Input: part model. Units: mm. Frame: model coordinates. A direction names the side the tool comes from. Give positions to 0.01 mm unless a question says otherwise; leave off trailing zeros. Write each loop counter-clockwise with the first axis right and the second up, starting at its lowest first coordinate (ties: lowest second). Pieces come first, ordered by that corner, then holes.
```python
from build123d import *

# Parameters (mm, degrees)
EXTRUDE_2_DEPTH     = 8
SKETCH_4_R          = 3.5
SKETCH_4_R_2        = 8.462893534
CUT_EXTRUDE_1_DEPTH = 126.60827275


with BuildPart() as part:
    # 草图1 → 凸台-拉伸2 (new body)
    with BuildSketch(Plane.XY):
        with BuildLine():
            ThreePointArc((-44.271832455, 12.900159535), (-42.760990151, 12.93891125), (-41.460762065, 13.709335217))
            ThreePointArc((-41.460762065, 13.709335217), (-27.63735599, 19.468755163), (-13.813949915, 13.709335217))
            ThreePointArc((-13.813949915, 13.709335217), (-12.513721829, 12.93891125), (-11.002879525, 12.900159535))
            Line((-11.002879525, 12.900159535), (59.529347881, 29.339622898))
            ThreePointArc((59.529347881, 29.339622898), (61.75543851, 28.989437599), (63.109724345, 27.188321525))
            Line((63.109724345, 27.188321525), (66.427142402, 14.703033787))
            ThreePointArc((66.427142402, 14.703033787), (65.985368626, 12.212155416), (63.796050229, 10.944668104))
            Line((63.796050229, 10.944668104), (-5.503908774, 4.721894109))
            ThreePointArc((-5.503908774, 4.721894109), (-7.526265644, 3.671148438), (-8.226657796, 1.502405805))
            ThreePointArc((-8.226657796, 1.502405805), (-8.168778443, 0.083161809), (-8.214531044, -1.33652486))
            ThreePointArc((-8.214531044, -1.33652486), (-7.503974356, -3.489473399), (-5.489913373, -4.530452062))
            Line((-5.489913373, -4.530452062), (63.846058336, -10.75645981))
            ThreePointArc((63.846058336, -10.75645981), (66.035376732, -12.023947122), (66.477150508, -14.514825493))
            Line((66.477150508, -14.514825493), (63.142843844, -27.063674443))
            ThreePointArc((63.142843844, -27.063674443), (61.732433193, -28.897690671), (59.436427456, -29.182701869))
            Line((59.436427456, -29.182701869), (-8.561409136, -10.190770239))
            ThreePointArc((-8.561409136, -10.190770239), (-10.364737659, -10.250456004), (-11.807672821, -11.33373541))
            ThreePointArc((-11.807672821, -11.33373541), (-27.63735599, -19.468755163), (-43.467039159, -11.33373541))
            ThreePointArc((-43.467039159, -11.33373541), (-44.909974321, -10.250456004), (-46.713302844, -10.190770239))
            Line((-46.713302844, -10.190770239), (-114.711139436, -29.182701869))
            ThreePointArc((-114.711139436, -29.182701869), (-117.007145173, -28.897690671), (-118.417555824, -27.063674443))
            Line((-118.417555824, -27.063674443), (-121.751862488, -14.514825493))
            ThreePointArc((-121.751862488, -14.514825493), (-121.310088712, -12.023947122), (-119.120770315, -10.75645981))
            Line((-119.120770315, -10.75645981), (-49.784798606, -4.530452062))
            ThreePointArc((-49.784798606, -4.530452062), (-47.770737623, -3.489473399), (-47.060180936, -1.33652486))
            ThreePointArc((-47.060180936, -1.33652486), (-47.105933537, 0.083161809), (-47.048054184, 1.502405805))
            ThreePointArc((-47.048054184, 1.502405805), (-47.748446336, 3.671148438), (-49.770803206, 4.721894109))
            Line((-49.770803206, 4.721894109), (-119.070762209, 10.944668104))
            ThreePointArc((-119.070762209, 10.944668104), (-121.260080606, 12.212155416), (-121.701854382, 14.703033787))
            Line((-121.701854382, 14.703033787), (-118.384436325, 27.188321525))
            ThreePointArc((-118.384436325, 27.188321525), (-117.03015049, 28.989437599), (-114.804059861, 29.339622898))
            Line((-114.804059861, 29.339622898), (-44.271832455, 12.900159535))
        make_face()
    extrude(amount=EXTRUDE_2_DEPTH)

    # 草图4 → 切除-拉伸1 (cut, through all)
    with BuildSketch(Plane.XY.offset(8)):
        with Locations((-115.63735599, -20)):
            Circle(SKETCH_4_R)
        with Locations((-115.63735599, 20)):
            Circle(SKETCH_4_R)
        with Locations((60.36264401, -20)):
            Circle(SKETCH_4_R)
        with Locations((60.36264401, 20)):
            Circle(SKETCH_4_R)
        with Locations((-27.63735599, 0)):
            Circle(SKETCH_4_R_2)
        with BuildLine():
            ThreePointArc((-37.984908909, -8.703484854), (-35.348611937, -6.039852319), (-38.012244471, -3.403555348))
            ThreePointArc((-38.012244471, -3.403555348), (-40.648541443, -6.067187882), (-37.984908909, -8.703484854))
        make_face()
        with BuildLine():
            ThreePointArc((-25.273693465, -13.312986121), (-26.26231842, -9.698069705), (-29.877234836, -10.68669466))
            ThreePointArc((-29.877234836, -10.68669466), (-28.888609881, -14.301611076), (-25.273693465, -13.312986121))
        make_face()
        with BuildLine():
            ThreePointArc((-19.502346355, -7.283139312), (-15.877424428, -8.234423195), (-14.926140546, -4.609501268))
            ThreePointArc((-14.926140546, -4.609501268), (-18.551062473, -3.658217385), (-19.502346355, -7.283139312))
        make_face()
        with BuildLine():
            ThreePointArc((-17.262467509, 3.403555348), (-14.626170537, 6.067187882), (-17.289803071, 8.703484854))
            ThreePointArc((-17.289803071, 8.703484854), (-19.926100043, 6.039852319), (-17.262467509, 3.403555348))
        make_face()
        with BuildLine():
            ThreePointArc((-25.397477144, 10.68669466), (-26.386102099, 14.301611076), (-30.001018515, 13.312986121))
            ThreePointArc((-30.001018515, 13.312986121), (-29.01239356, 9.698069705), (-25.397477144, 10.68669466))
        make_face()
        with BuildLine():
            ThreePointArc((-35.772365625, 7.283139312), (-39.397287552, 8.234423195), (-40.348571434, 4.609501268))
            ThreePointArc((-40.348571434, 4.609501268), (-36.723649507, 3.658217385), (-35.772365625, 7.283139312))
        make_face()
    extrude(amount=-CUT_EXTRUDE_1_DEPTH, mode=Mode.SUBTRACT)


solid = part.part
```
Item 1: Set-up query: faces 4 (the cylindrical face through (-19.82, -3.24, 4.06)), 5 (the flat face through (-84.938, -7.687, 3.944)), 6 (the flat face through (28.7, -7.6, 3.9)), 7 (the flat face through (-120.06, -20.88, 3.94)), 8 (the flat face through (23.77, 21.005, 3.944)). Return all of +Z, -Z, +X, -X, +Y, -Y with unobstructed straight access to the full face (end or side cutting, diameter ignored); none if empty.
Item 2: Section B-B (x = 28.5). Return loops of the section in (y, z), and give its area (3 significant figures).
Item 3: Mould query, pull axis X, two halves, no side actions, for faces 1 (the flat face through (64.745, 21.033, 3.944)), 2 (the flat face through (-120.066, 20.858, 3.944)), 3 (the cylindrical face through (59.91, -16.53, 4.06)). Classes: +X half, -X half, draft (parallel to the pull), parting line (faces both ways), or undercut.
Item 4: Section C-C (z = 4). Give the number of separate pieces and of enclosed holes in the cut face, and give its area (3 significant figures).
Item 5: Ray query, line 1 (Y direction, x = -36.5, z = 2.5); line 2 (X direction, y = -2.5, z = 5.5); line 3 (Y direction, x = 30.5, z = 2.5). Return the intervals inside material, ascending.
Item 6: Section A-A (x = -101.5). Return loops of the section in (y, z), and give its area (3 significant figures).
Item 7: Pin query (flat end, axial travel): pin 1 (4 mm diameter, centred on x = -27.58, y = -12, fed in from -Z); pin 2 (4 mm diameter, centred on y = -19, z = 1.5, fed in from +X); pin 3 (3 mm diameter, centred on x = -50.5, z = 4.5, fed in from +Y). Return the tip coordinate at first contact, or that it passes through.
Solved:
1. face 4: +Z, -Z
1. face 5: +Z, -Z, -X
1. face 6: +Z, -Z, +X
1. face 7: +Z, -Z, -X, -Y
1. face 8: +Z, -Z, +Y
2. outline: (-20.54, 0) - (-7.58, 0) - (-7.58, 8) - (-20.54, 8) - close; (7.78, 0) - (22.11, 0) - (22.11, 8) - (7.78, 8) - close
2. area: 218 mm2
3. face 1: +X half
3. face 2: -X half
3. face 3: undercut
4. separate pieces: 1
4. enclosed holes: 11
4. area: 4,700 mm2
5. line 1: y = -17.33 to -8.24, -3.87 to 3.8, 8.09 to 17.33
5. line 2: x = -47.21 to -35.72, -19.55 to -8.06
5. line 3: y = -21.1 to -7.76, 7.95 to 22.57
6. outline: (-25.49, 0) - (-9.17, 0) - (-9.17, 8) - (-25.49, 8) - close; (9.37, 0) - (26.24, 0) - (26.24, 8) - (9.37, 8) - close
6. area: 266 mm2
7. pin 1: passes through
7. pin 2: stops at x = 65.82
7. pin 3: stops at y = 14.7
